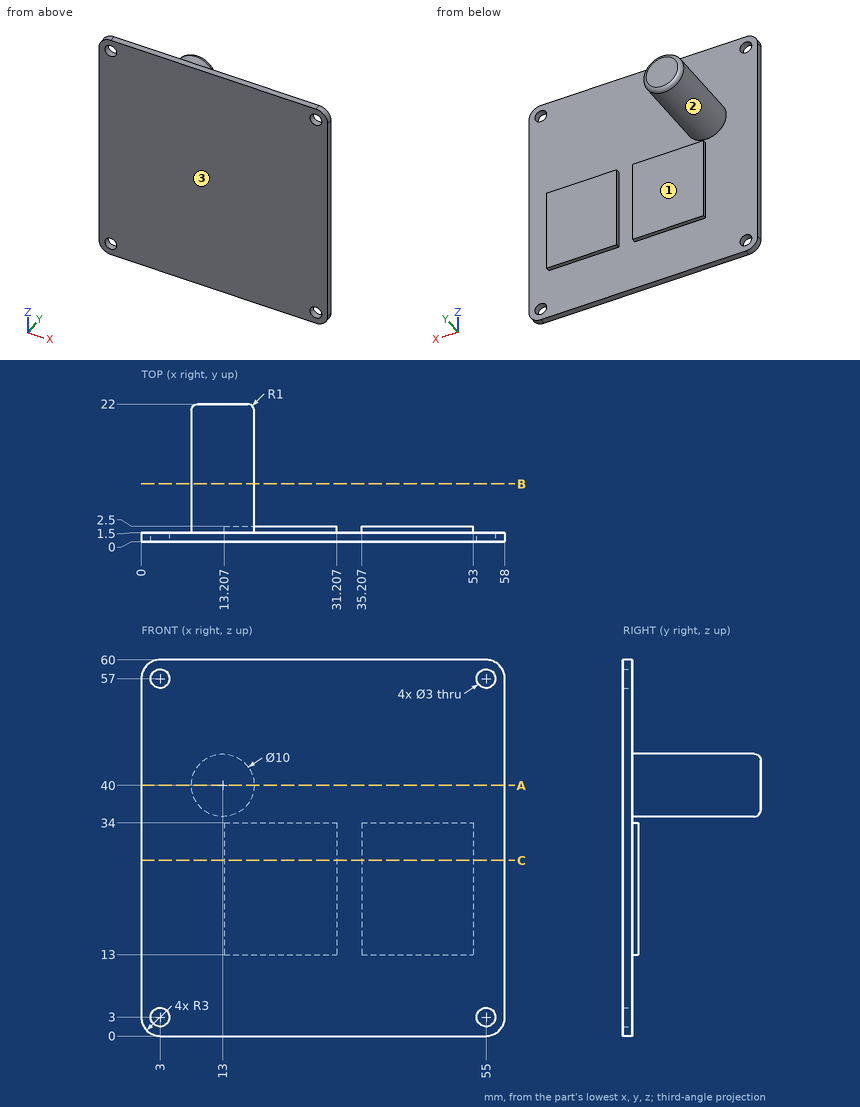
Drawing for the job (mm, zero at the part's lowest x, y, z). A direction names the side the tool comes from. Give positions to 0.01 mm unless a question says otherwise; leave off trailing zeros. Loops run counter-clockwise (first coordinate to the right, second up) from the corner with the lowest first, then second, coordinate; pieces in that order, holes last.
1) Drop flat-ended pins along their axis: P1, Ø2, axis at y = 13, z = 45, coming from the -X side; P2, Ø5, axis at x = 3, z = 57, coming from the +Y side; P3, Ø5.5, axis at x = 47.5, z = 20.5, coming from the +Y side. Give the stop position or say it passes through.
Values follow:
P1: stops at x = 10
P2: stops at y = 1.5
P3: stops at y = 2.5
2) Band-saw the part on A-A on z = 40. List the corners of the cut face in (x, y).
Values follow:
outline: (0, 0) - (58, 0) - (58, 1.5) - (18, 1.5) - (18, 21) arc R1 ccw to (17, 22) - (9, 22) arc R1 ccw to (8, 21) - (8, 1.5) - (0, 1.5) - close
3) Probe line 1 along X through (y, z) = (0.5, 3); line 2 along Z through (x, y) = (55, 1.1); line 3 along Y through (x, z) = (24, 54). List the from-to ranges inside material, lowest first.
Values follow:
line 1: x = 0 to 1.5, 4.5 to 53.5, 56.5 to 58
line 2: z = 0 to 1.5, 4.5 to 55.5, 58.5 to 60
line 3: y = 0 to 1.5
4) Band-saw the part on B-B on y = 9.25. List the corners of the cut face in (x, z).
Values follow:
outline: circle Ø10 at (13, 40)
5) Band-saw the part on C-C on z = 28. List the corners of the cut face in (x, y), then the cut area to 3 significant figures.
Values follow:
outline: (0, 0) - (58, 0) - (58, 1.5) - (53, 1.5) - (53, 2.5) - (35.21, 2.5) - (35.21, 1.5) - (31.21, 1.5) - (31.21, 2.5) - (13.21, 2.5) - (13.21, 1.5) - (0, 1.5) - close
area: 123 mm2
6) 3-axis set-ups, long thin cutter, end or side, ignore diameter. For the marked faces 1, 2 and 3: which of +Z, -Z, +X, -X, +Y, -Y reach the whole face in a straight line?
Values follow:
face 1: -Z, +X, -X, +Y
face 2: +Y
face 3: +Z, -Z, +X, -X, -Y
